Read the model definition and answer for the solid it produces. Units are mm, in the model's axes. A direction names the side the tool comes from. Round coordinates to 2 decimals unless told otherwise and drop trailing zeros. Answer as CSV lines item,"result".
```python
from build123d import *

# Parameters (mm, degrees)
BOSS_EXTRUDE1_DEPTH   = 6
FILLET3_R             = 3
F_4_40_TAPPED_HOLE1_D = 2.2606
F_4_40_TAPPED_HOLE2_D = 2.2606
F_4_40_TAPPED_HOLE3_D = 2.2606


with BuildPart() as part:
    # Sketch1 → Boss-Extrude1 (new body)
    with BuildSketch(Plane(origin=(0, 0, 0), x_dir=(1, 0, 0), z_dir=(0, 1, 0))):
        Polygon((-24.694969511, -1.227058116), (-11.284821255, 22), (-25, 22), (-25, 28), (25, 28), (25, 22), (11.284821255, 22), (24.694969511, -1.227058116), (31.552558883, 10.650635095), (36.748711306, 7.650635095), (11.748711306, -35.650635095), (6.552558883, -32.650635095), (13.410148256, -20.772941884), (-13.410148256, -20.772941884), (-6.552558883, -32.650635095), (-11.748711306, -35.650635095), (-36.748711306, 7.650635095), (-31.552558883, 10.650635095), align=None)
    extrude(amount=BOSS_EXTRUDE1_DEPTH)

    # Fillet3
    fillet3_edges = [part.edges().sort_by_distance(p)[0] for p in [
        (24.248711306, 0, 14),
        (24.248711306, 6, 14),
        (0, 0, -28),
        (0, 6, -28),
        (-24.248711306, 0, 14),
        (-24.248711306, 6, 14),
        (9.981353569, 0, 26.711788489),
        (9.981353569, 6, 26.711788489),
        (28.123764197, 0, -4.711788489),
        (28.123764197, 6, -4.711788489),
        (18.142410628, 0, -22),
        (18.142410628, 6, -22),
        (-18.142410628, 6, -22),
        (-18.142410628, 0, -22),
        (-28.123764197, 6, -4.711788489),
        (-28.123764197, 0, -4.711788489),
        (-9.981353569, 0, 26.711788489),
        (-9.981353569, 6, 26.711788489),
    ]]
    fillet(fillet3_edges, radius=FILLET3_R - 0.0001)  # a hair under: the kernel refuses the full size

    # #4-40 Tapped Hole1 (through all)
    with Locations(Plane(origin=(12.5, 0, 21.650635095), x_dir=(0.866025403784438, 0, -0.5000000000000012), z_dir=(0.5000000000000012, 0, 0.866025403784438))):
        with Locations((-25, 3)):
            Hole(F_4_40_TAPPED_HOLE1_D / 2)

    # #4-40 Tapped Hole2 (through all)
    with Locations(Plane(origin=(12.5, 0, -21.650635095), x_dir=(-0.8660254037844389, 0, -0.4999999999999995), z_dir=(0.4999999999999995, 0, -0.8660254037844389))):
        with Locations((-25, 3)):
            Hole(F_4_40_TAPPED_HOLE2_D / 2)

    # #4-40 Tapped Hole3 (through all)
    with Locations(Plane.ZY.offset(25)):
        with Locations((-25, 3)):
            Hole(F_4_40_TAPPED_HOLE3_D / 2)


solid = part.part
```
1) A cutting plane is placed at B-B, the plane z = -6.5. Count the separate pieces of the cut face and the enclosed holes in it, plus the area to 3 significant figures.
Entries:
separate pieces,"3"
enclosed holes,"2"
area,"299 mm^2"
2) The mould has two halves that part along Z. Classify faces 4 (the face through (17.17, 5.1, -22.86)), 5 (the face through (0, 6, -2)), 6 (the face through (-11.101, 5.098, 26.483)), 7 (the face through (9.187, 4.291, 34.172)): pulls with the +Z half, pulls with the -Z half, needs draft (parallel to the pull), parting line crosses it, or undercut.
Entries:
face 4,"undercut"
face 5,"needs draft"
face 6,"undercut"
face 7,"pulls with the +Z half"
3) Each of these flat-tipped pins is pushed along its axis until it touches: P1, Ø6, axis at x = 21, z = 25, coming from the -Y side; P2, Ø10, axis at x = -19.5, z = 22, coming from the +Y side; P3, Ø1, axis at x = 13.5, y = 2.5, coming from the +Z side. Where does it stop, or does it pass through?
Entries:
P1,"stops at y = 1.66"
P2,"stops at y = 6"
P3,"stops at z = 33.41"
4) A tool of negligible diameter and unlimited length cuts with its end or side. For faces 1 (the face through (25, 3, -23.7)), 2 (the face through (-17.38, 0.9, -22.86)), 3 (the face through (-9.114, 4.291, 34.13)), from which of +Z, -Z, +X, -X, +Y, -Y can it reach the whole face along a straight path? Write none if from no direction.
Entries:
face 1,"-Z, +X, +Y, -Y"
face 2,"-X, -Y"
face 3,"+Z, +Y, -Y"
5) Find the intervals of material crossed by line 1 (Z direction, x = 12, y = 4.3); line 2 (Y direction, x = 6.5, z = -25); line 3 (X direction, y = 2.2, z = -5), in increasing order.
Entries:
line 1,"z = -27.7 to -22.3, -20.76 to 20.77, 23.81 to 34.62"
line 2,"y = 0 to 1.87, 4.13 to 6"
line 3,"x = -35.09 to -32.68, -30.83 to -28.42, -21.1 to 21.1, 28.42 to 30.83, 32.68 to 35.09"
